Verification items for the finished model (mm, model axes). A direction names the side the tool comes from. Give positions to 0.01 mm unless a question says otherwise; leave off trailing zeros. Write each loop counter-clockwise with the first axis right and the second up, starting at its lowest first coordinate (ties: lowest second). Pieces come first, ordered by that corner, then holes. Notation, with made-up numbers: M 64,6 L 101,6 A20 cw 101,14 Z; hole C -1,54 d4. An arc over 180 degrees is marked long. Answer as a JSON object with one key per item and string values.
```python
from build123d import *

# Parameters (mm, degrees)
F0_R     = 3.175
F1_DEPTH = 9.525
F0_R_2   = 12.7
F2_DEPTH = 6.35


# Not quite as in the source:
# - a feature of the source that left no trace in its solid (it failed there, or was rolled back) is left out


with BuildPart() as f1:
    # F0 (on Right) → F1 (new body, symmetric)
    with BuildSketch(Plane.YZ):
        Circle(F0_R)
    extrude(amount=F1_DEPTH, both=True)

    # F0 (on Right) → F2 (join, symmetric)
    with BuildSketch(Plane.YZ):
        Circle(F0_R_2)
        Circle(F0_R, mode=Mode.SUBTRACT)
    extrude(amount=F2_DEPTH, both=True)


solid = f1.part
```
1) Section check D-D on x = 7.75. Record the boundary of the cut face in (y, z) (3 decimals).
Completed:
{"outline": "C 0,0 d6.35"}
2) Go/stop test with flat-tipped pins: pin 1 (12.5 mm diameter, centred on y = 5.5, z = -1, fed in from +X) (3 decimals); pin 2 (6 mm diameter, centred on x = -3.5, z = 8.5, fed in from -Y); pin 3 (1.5 mm diameter, centred on x = -4.5, z = 2.5, fed in from +Y); pin 4 (3 mm diameter, centred on x = -3, y = 9, fed in from +Z). Record where each tip stops, or that it passes through.
Completed:
{"pin 1": "stops at x = 9.525", "pin 2": "stops at y = -11.45", "pin 3": "stops at y = 12.58", "pin 4": "stops at z = 10.25"}
3) Access from +Z, -Z, +X, -X, +Y, -Y to the whole of each face (thin tool, end or side, straight path). Record for faces 1 (the face through (-7.92, -0.69, -3.1)), 2 (the face through (6.35, 3, -3)), 3 (the face through (0.09, -2.75, -12.4)).
Completed:
{"face 1": "-X", "face 2": "+X", "face 3": "+X, -X"}
4) Section check A-A on y = 0. Record the boundary of the cut face in (x, z) (3 decimals), and give its area (3 significant figures).
Completed:
{"outline": "M -9.525,-3.175 L -6.35,-3.175 L -6.35,-12.7 L 6.35,-12.7 L 6.35,-3.175 L 9.525,-3.175 L 9.525,3.175 L 6.35,3.175 L 6.35,12.7 L -6.35,12.7 L -6.35,3.175 L -9.525,3.175 Z", "area": "363 mm2"}
5) Thickness scan on L1, parallel to X at y = 5, z = -6; L2, parallel to Z at x = -3, y = 2; L3, parallel to Y at x = -1.75, z = -10.75. Record the ranges inside material, lowest first.
Completed:
{"L1": "x = -6.35 to 6.35", "L2": "z = -12.54 to 12.54", "L3": "y = -6.76 to 6.76"}
6) Section check B-B on x = -0.5. Record the boundary of the cut face in (y, z).
Completed:
{"outline": "C 0,0 d25.4"}
7) Section check C-C on z = 5.25. Record the boundary of the cut face in (x, y), and give its area (3 significant figures).
Completed:
{"outline": "M -6.35,-11.56 L 6.35,-11.56 L 6.35,11.56 L -6.35,11.56 Z", "area": "294 mm2"}
